from build123d import *

# Parameters (mm, degrees)
BOSS_EXTRUDE1_DEPTH = 7


with BuildPart() as part:
    # Sketch1 → Base-Revolve (revolve)
    with BuildSketch(Plane(origin=(0, 0, 0), x_dir=(1, 0, 0), z_dir=(0, 1, 0))):
        Polygon((0, 0), (0, -20), (3.5, -20), (3.5, -15), (5, -15), (5, 0), align=None)
    revolve(axis=Axis((0, 0, -1.187299328), (0, 0, 1)))

    # Sketch2 → Boss-Extrude1 (add)
    with BuildSketch(Plane(origin=(0, 0, 0), x_dir=(-1, 0, 0), z_dir=(0, 0, -1))):
        Polygon((6, -3.464101615), (6, 3.464101615), (0, 6.92820323), (-6, 3.464101615), (-6, -3.464101615), (0, -6.92820323), align=None)
    extrude(amount=BOSS_EXTRUDE1_DEPTH)


solid = part.part
Can you work these out from the model? Positions are in its coordinate system, mm. A direction names the side the tool comes from. Coordinates: 2 decimals unless noted, no trailing zeros. Write each loop counter-clockwise with the first axis right and the second up, starting at its lowest first coordinate (ties: lowest second). Pieces come first, ordered by that corner, then holes.
Q1. Imagine slicing it at A-A, the plane y = 0. List the corners of the cut face in (x, z) for me, plus the area to 3 significant figures.
Results found:
outline: (-6, -7) - (6, -7) - (6, 0) - (5, 0) - (5, 15) - (3.5, 15) - (3.5, 20) - (-3.5, 20) - (-3.5, 15) - (-5, 15) - (-5, 0) - (-6, 0) - close
area: 269 mm2
Q2. Imagine slicing it at D-D, the plane x = -4.5. List the corners of the cut face in (y, z) for me.
Results found:
outline: (-4.33, -7) - (4.33, -7) - (4.33, 0) - (2.18, 0) - (2.18, 15) - (-2.18, 15) - (-2.18, 0) - (-4.33, 0) - close
Q3. Imagine slicing it at C-C, the plane z = 3.5. List the corners of the cut face in (x, y) for me.
Results found:
outline: circle Ø10 at (0, 0)
Q4. Please list where these lines run through material, in increasing order: L1, parallel to Z at x = -4.5, y = 4.25; L2, parallel to Z at x = 4, y = -2; L3, parallel to Y at x = 0.5, z = 5.
Results found:
L1: z = -7 to 0
L2: z = -7 to 15
L3: y = -4.97 to 4.97
Q5. Which directions (+Z, -Z, +X, -X, +Y, -Y) give clear straight access to the entire face, cutting with the end or side of a thin tool? Please do faces 1 (the face through (-2.96, -5.22, -3.45)), 2 (the face through (-2.2, -3.3, 15)).
Results found:
face 1: +Z, -Z, -X, -Y
face 2: +Z
Q6. Imagine slicing it at B-B, the plane x = 2.5. List the corners of the cut face in (y, z) for me, plus the area to 3 significant figures.
Results found:
outline: (-5.48, -7) - (5.48, -7) - (5.48, 0) - (4.33, 0) - (4.33, 15) - (2.45, 15) - (2.45, 20) - (-2.45, 20) - (-2.45, 15) - (-4.33, 15) - (-4.33, 0) - (-5.48, 0) - close
area: 231 mm2
Q7. For P1, Ø3, axis at x = 2, z = 10, coming from the -Y side; P2, Ø6, axis at x = 4, y = 1.5, coming from the +Z side; P3, Ø2, axis at x = 4.5, y = 5, coming from the +Z side, each with a flat end and sliding along its axis, tell me the tip position at first contact or that it passes through.
Results found:
P1: stops at y = -4.97
P2: stops at z = 20
P3: stops at z = 0
